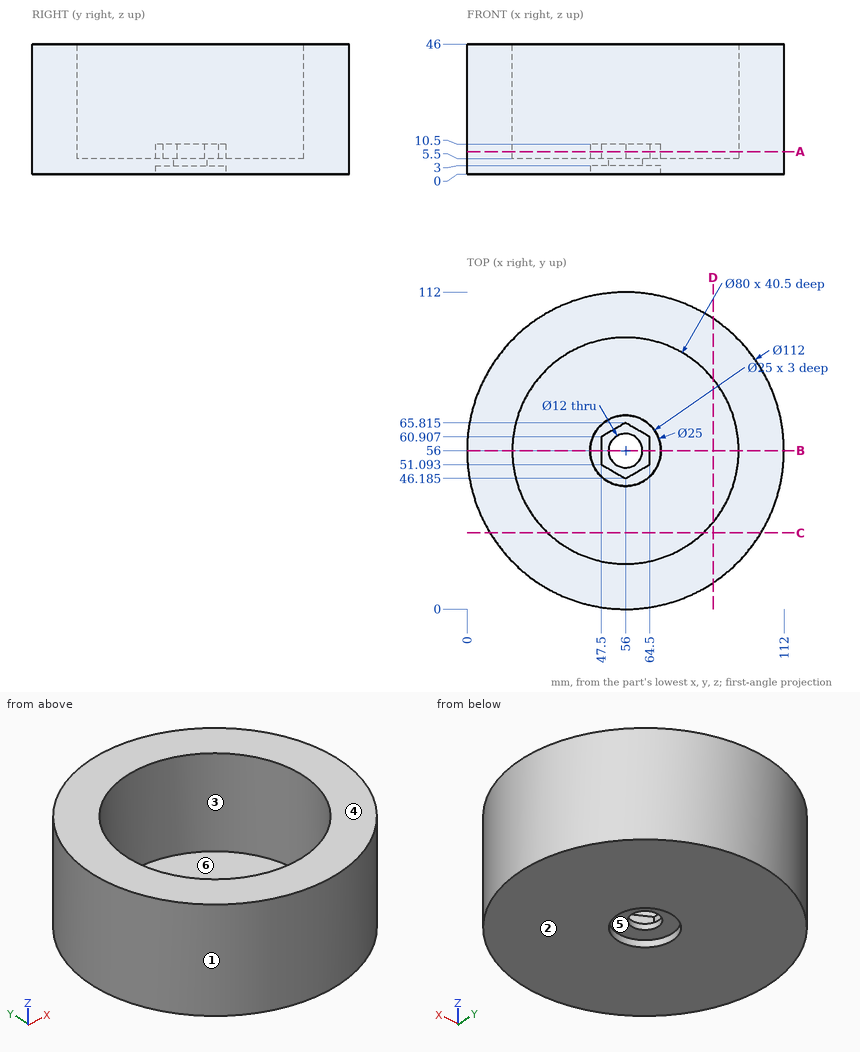
Geometry check sheet. Reference: drawing and pictorial views, mm from the part's lowest x, y, z. A direction names the side the tool comes from. Give positions to 0.01 mm unless a question says otherwise; leave off trailing zeros. Order: outer loops, then holes, each group sorted by start corner. A loop starts at its lowest first (then second) coordinate and runs counter-clockwise, first axis right, second up. Notation, with made-up numbers: (4, 16) -> (44, 16) arc R25 cw to (44, 32) -> close; hole circle Ø1 at (-1, 34.5). An arc over 180 degrees is marked (long way). Use CSV: the item, a comma, the result in double quotes. Start each with the question number.
1) Material ranges on line 1 (Y direction, x = 56, z = 2); line 2 (Y direction, x = 56, z = 32); line 3 (Z direction, x = 23, y = 77.5), recorded low to high. Write a range as from..to.
2) Go/stop test with flat-tipped pins: P1, Ø3, axis at x = 25.5, z = 31, coming from the -Y side (1 decimal); P2, Ø4, axis at x = 29.5, y = 79, coming from the +Z side; P3, Ø1.5, axis at y = 58, z = 8.5, coming from the -X side; P4, Ø2.5, axis at y = 55, z = 7, coming from the +X side. Record where each tip stops, or that it passes through.
3) Mould release check, pull along X, two halves, no side actions. Record for the marked faces 1, 2 and 3: released by +X, released by -X, zero draft, split by the parting line, or undercut.
4) Set-up check for the marked faces 4, 5 and 6: record each of +Z, -Z, +X, -X, +Y, -Y from which the full face is reachable in a straight line by a thin tool's end or side.
5) Sectioned sample at D-D, the plane x = 87. Record the boundary of the cut face in (y, z).
6) Sectioned sample at B-B, the plane y = 56. Record the boundary of the cut face in (x, z), plus the area to 3 significant figures.
7) Sectioned sample at A-A, the plane z = 8. Record the boundary of the cut face in (x, y) (1 decimal).
8) Sectioned sample at C-C, the plane y = 27. Record the boundary of the cut face in (x, z).
Recorded:
1,line 1,"0..43.5, 68.5..112"
1,line 2,"0..16, 96..112"
1,line 3,"0..5.5"
2,P1,"y = 8.1"
2,P2,"z = 5.5"
2,P3,"x = 0.01"
2,P4,"x = 112"
3,face 1,"split by the parting line"
3,face 2,"zero draft"
3,face 3,"undercut"
4,face 4,"+Z, +X, -X, +Y, -Y"
4,face 5,"-Z"
4,face 6,"+Z"
5,outline,"(9.36, 0) -> (102.64, 0) -> (102.64, 46) -> (81.28, 46) -> (81.28, 5.5) -> (30.72, 5.5) -> (30.72, 46) -> (9.36, 46) -> close"
6,outline,"(0, 0) -> (43.5, 0) -> (43.5, 3) -> (50, 3) -> (50, 5.5) -> (47.5, 5.5) -> (47.5, 10.5) -> (43.5, 10.5) -> (43.5, 5.5) -> (16, 5.5) -> (16, 46) -> (0, 46) -> close; (62, 3) -> (68.5, 3) -> (68.5, 0) -> (112, 0) -> (112, 46) -> (96, 46) -> (96, 5.5) -> (68.5, 5.5) -> (68.5, 10.5) -> (64.5, 10.5) -> (64.5, 5.5) -> (62, 5.5) -> close"
6,area,"1,850 mm2"
7,outline,"circle Ø112 at (56, 56); circle Ø25 at (56, 56); hole circle Ø80 at (56, 56); hole (47.5, 51.1) -> (56, 46.2) -> (64.5, 51.1) -> (64.5, 60.9) -> (56, 65.8) -> (47.5, 60.9) -> close"
8,outline,"(8.09, 0) -> (103.91, 0) -> (103.91, 46) -> (83.55, 46) -> (83.55, 5.5) -> (28.45, 5.5) -> (28.45, 46) -> (8.09, 46) -> close"
